The listing builds one solid part. Answer for the finished solid, in the listing's coordinates (mm). A direction names the side the tool comes from. Give positions to 0.01 mm unless a question says otherwise; leave off trailing zeros. Write each loop counter-clockwise with the first axis right and the second up, starting at its lowest first coordinate (ties: lowest second). Pieces come first, ordered by that corner, then holes. Notation, with made-up numbers: (2.25, 12.25) - (12.25, 12.25) arc R25 ccw to (12.25, 30.25) - close; hole circle Ø3 at (55, 9.25). An arc over 180 degrees is marked (long way). Use a Markdown table: item, result. Add a question column.
from build123d import *

# Parameters (mm, degrees)
F0_W     = 609.6
F0_H     = 88.9
F1_DEPTH = 38.1
F2_R     = 6.35
F5_DEPTH = 76.2
F3_R     = 6.35
F4_DEPTH = 76.2
F6_R     = 6.35


with BuildPart() as f1:
    # F0 (on Front) → F1 (new body)
    with BuildSketch(Plane.XZ):
        with Locations((0, -23.109551)):
            Rectangle(F0_W, F0_H)
    extrude(amount=-F1_DEPTH)

    # F2 (on face) → F5 (cut)
    with BuildSketch(Plane(origin=(-304.8, 0, 0), x_dir=(0, -1, 0), z_dir=(-1, 0, 0))):
        with Locations((-19.05, -8.377551)):
            Circle(F2_R)
        with Locations((-19.05, -37.841551)):
            Circle(F2_R)
    extrude(amount=-F5_DEPTH, mode=Mode.SUBTRACT)

    # F3 (on face) → F4 (cut)
    with BuildSketch(Plane.YZ.offset(304.8)):
        with Locations((19.05, -8.377551)):
            Circle(F3_R)
        with Locations((19.05, -37.841551)):
            Circle(F3_R)
    extrude(amount=-F4_DEPTH, mode=Mode.SUBTRACT)

    # F6
    f6_edges = [f1.edges().sort_by_distance(p)[0] for p in [
        (0, 0, 21.340449),
        (0, 38.1, 21.340449),
        (0, 38.1, -67.559551),
        (0, 0, -67.559551),
    ]]
    fillet(f6_edges, radius=F6_R)


solid = f1.part
1. The part is cut by section A-A (y = 19.05). Give the vertices of the cut face in (x, z).
2. For a pull along Y with two mould halves and no side action, classify faces 1 (the flat face through (-4, 19, -67.56)), 2 (the flat face through (-4, 0, -23)), 3 (the cylindrical face through (267.233, 25.107, -35.934)) as released by +Y, released by -Y, zero draft, split by the parting line, or undercut.
3. Which of the six approach directions +Z, -Z, +X, -X, +Y, -Y give full straight-line access (tool end or side, diameter ignored) to faces 4 (the flat face through (304.8, 19, -24)), 5 (the cylindrical face through (267.233, 25.107, -6.47)), 6 (the cylindrical face through (-267.233, 25.394, -37.562))?
4. Given P1, Ø7.5, axis at y = 19.05, z = -8.38, coming from the +X side; P2, Ø6.5, axis at y = 21, z = -37, coming from the -X side, each flat-ended and moving along its own axis, determine where each tip first touches the part or whether it passes through.
5. Consider L1, parallel to Z at x = 287, y = 19.05; L2, parallel to X at y = 23, z = -8; L3, parallel to Y at x = 188.5, z = -62. Determine where each line is inside the solid, lowest interval first. Write a range as [from, to].
Check values:
| question | item | result |
|---|---|---|
| 1 | outline | (-304.8, -67.56) - (304.8, -67.56) - (304.8, -44.19) - (228.6, -44.19) - (228.6, -31.49) - (304.8, -31.49) - (304.8, -14.73) - (228.6, -14.73) - (228.6, -2.03) - (304.8, -2.03) - (304.8, 21.34) - (-304.8, 21.34) - (-304.8, -2.03) - (-228.6, -2.03) - (-228.6, -14.73) - (-304.8, -14.73) - (-304.8, -31.49) - (-228.6, -31.49) - (-228.6, -44.19) - (-304.8, -44.19) - close |
| 2 | face 1 | zero draft |
| 2 | face 2 | released by -Y |
| 2 | face 3 | undercut |
| 3 | face 4 | +Z, -Z, +X, +Y, -Y |
| 3 | face 5 | +X |
| 3 | face 6 | -X |
| 4 | P1 | stops at x = 228.6 |
| 4 | P2 | stops at x = -228.6 |
| 5 | L1 | z = [-67.56, -44.19], [-31.49, -14.73], [-2.03, 21.34] |
| 5 | L2 | x = [-228.6, 228.6] |
| 5 | L3 | y = [0.05, 38.05] |
